```python
from build123d import *

# Parameters (mm, degrees)
BOSS_EXTRUDE1_DEPTH = 66
CUT_EXTRUDE1_START  = -3
SKETCH2_W           = 15
SKETCH2_H           = 50
CUT_EXTRUDE1_DEPTH  = 60
SKETCH3_W           = 32
SKETCH3_H           = 38
CUT_EXTRUDE2_DEPTH  = 19
SKETCH4_R           = 4
SKETCH4_R_2         = 2
CUT_EXTRUDE3_DEPTH  = 22


with BuildPart() as part:
    # Sketch1 → Boss-Extrude1 (new body)
    with BuildSketch(Plane(origin=(0, 0, 0), x_dir=(0, 0, -1), z_dir=(1, 0, 0))):
        Polygon((-3, -25.9), (-21, -25.9), (-21, -85.9), (0, -85.9), (0, 0), (-3, 0), align=None)
    extrude(amount=-BOSS_EXTRUDE1_DEPTH)

    # Sketch2 → Cut-Extrude1 (cut)
    with BuildSketch(Plane(origin=(0, 0, 0), x_dir=(0, 0, -1), z_dir=(1, 0, 0)).offset(CUT_EXTRUDE1_START)):
        with Locations((-10.5, -50.9)):
            Rectangle(SKETCH2_W, SKETCH2_H)
    extrude(amount=-CUT_EXTRUDE1_DEPTH, mode=Mode.SUBTRACT)

    # Sketch3 → Cut-Extrude2 (cut, through all)
    with BuildSketch(Plane.XY.offset(3)):
        with Locations((-33, -44.9)):
            Rectangle(SKETCH3_W, SKETCH3_H)
    extrude(amount=CUT_EXTRUDE2_DEPTH, mode=Mode.SUBTRACT)

    # Sketch4 → Cut-Extrude3 (cut, through all)
    with BuildSketch(Plane(origin=(0, 0, 0), x_dir=(-1, 0, 0), z_dir=(0, 0, -1))):
        with Locations((33, -47.9)):
            Circle(SKETCH4_R)
        with Locations((33, -80.9)):
            Circle(SKETCH4_R_2)
        with Locations((58, -8)):
            Circle(SKETCH4_R_2)
        with Locations((8, -8)):
            Circle(SKETCH4_R_2)
    extrude(amount=-CUT_EXTRUDE3_DEPTH, mode=Mode.SUBTRACT)


solid = part.part
```
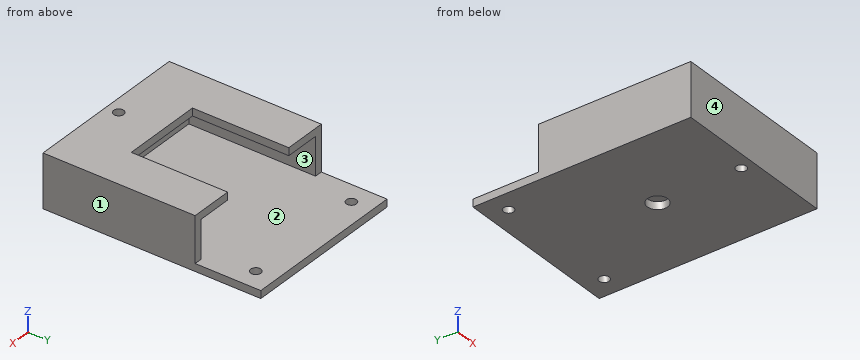
Work out the finished part from the listing and answer in its coordinate system (mm). Face numbers are marked on the shaded views. Coordinates: 2 decimals unless noted, no trailing zeros. Write each loop counter-clockwise with the first axis right and the second up, starting at its lowest first coordinate (ties: lowest second). Pieces come first, ordered by that corner, then holes. Notation, with made-up numbers: (15.25, 15.25) - (42.25, 15.25) arc R17 ccw to (42.25, 30.25) - close; hole circle Ø9 at (24, -37). An arc over 180 degrees is marked (long way). Answer as a JSON object with one key per item and string values.
Q1. Consider L1, parallel to X at y = -46.5, z = 7.5; L2, parallel to Z at x = -5, y = -49.5; L3, parallel to Y at x = -8, z = 2.35. Determine where each line is inside the solid, lowest interval first. Write a range as from..to.
Results list:
{"L1": "x = -66..-63, -3..0", "L2": "z = 0..3, 18..21", "L3": "y = -85.9..-10, -6..0"}
Q2. Find section C-C (y = -80.9). Write down the section's boundary in (x, z).
Results list:
{"outline": "(-66, 0) - (-35, 0) - (-35, 21) - (-66, 21) - close; (-31, 0) - (0, 0) - (0, 21) - (-31, 21) - close"}
Q3. For a pull along X with two mould halves and no side action, classify the marked faces 1, 2, 3 and 4 as pulls with the +X half, pulls with the -X half, needs draft (parallel to the pull), parting line crosses it, or undercut.
Results list:
{"face 1": "pulls with the +X half", "face 2": "undercut", "face 3": "undercut", "face 4": "needs draft"}
Q4. Find section B-B (y = -8). Write down the section's boundary in (x, z).
Results list:
{"outline": "(-66, 0) - (-60, 0) - (-60, 3) - (-66, 3) - close; (-56, 0) - (-10, 0) - (-10, 3) - (-56, 3) - close; (-6, 0) - (0, 0) - (0, 3) - (-6, 3) - close"}
Q5. Given pin 1 Ø3 at (x, y) = (-33, -80.9) entering from +Z; pin 2 Ø5 at (x, y) = (-16.5, -10.5) entering from +Z; pin 3 Ø4.5 at (x, z) = (-29, 8) entering from +Y; pin 4 Ø8.5 at (x, z) = (-54.5, 16.5) entering from +Y, each flat-ended and moving along its own axis, determine where each tip first touches the part or whether it passes through.
Results list:
{"pin 1": "passes through", "pin 2": "stops at z = 3", "pin 3": "stops at y = -75.9", "pin 4": "stops at y = -25.9"}
Q6. Find section D-D (x = -41). Write down the section's boundary in (y, z).
Results list:
{"outline": "(-85.9, 0) - (0, 0) - (0, 3) - (-75.9, 3) - (-75.9, 18) - (-63.9, 18) - (-63.9, 21) - (-85.9, 21) - close"}
Q7. Find section A-A (x = -58). Write down the section's boundary in (y, z), plus the area to 3 significant figures.
Results list:
{"outline": "(-85.9, 0) - (-10, 0) - (-10, 3) - (-75.9, 3) - (-75.9, 18) - (-25.9, 18) - (-25.9, 21) - (-85.9, 21) - close; (-6, 0) - (0, 0) - (0, 3) - (-6, 3) - close", "area": "576 mm^2"}
